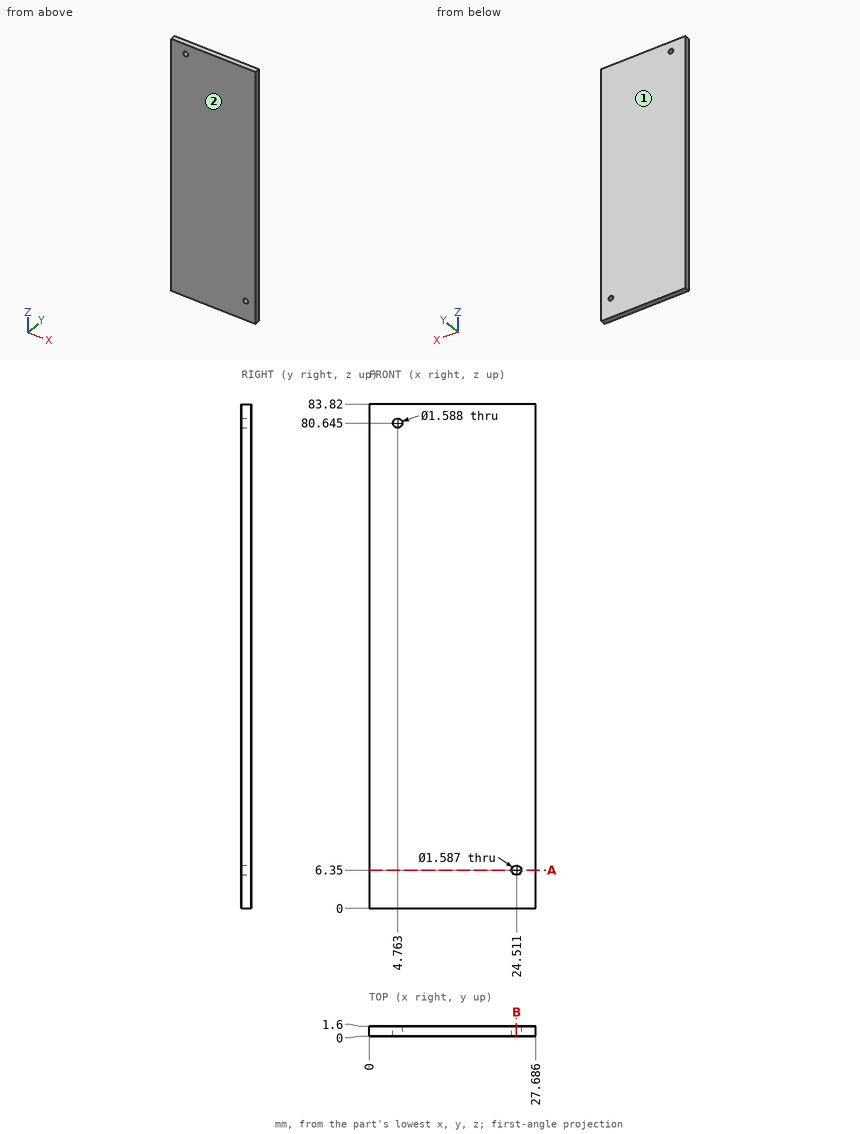
Here's the drawing with two shaded views (mm, measured from the low corner). I have some questions. Coordinates: 2 decimals unless noted, no trailing zeros. Write each loop counter-clockwise with the first axis right and the second up, starting at its lowest first coordinate (ties: lowest second). Pieces come first, ordered by that corner, then holes. Notation, with made-up numbers: M 5.25,-31 L 15.25,-31 A32 ccw 15.25,-5 Z; hole C -4,81.5 d4. An arc over 180 degrees is marked long. Answer as CSV lines item,"result". Start each with the question number.
1) I want a section at A-A, the plane z = 6.35. Please give me the cut outline in (x, y) (1 decimal).
2) We'd pull the mould along Y, two halves only. Please class the marked faces 1 and 2: +Y half, -Y half, draft (parallel to the pull), parting line (faces both ways), or undercut.
3) Please list where this line runs through material, in increasing order: line 1 (X direction, y = 0.2, z = 6) (1 decimal). Write a range as from..to.
4) I want a section at B-B, the plane x = 24.5. Please give me the cut outline in (y, z).
Data:
1,outline,"M 0,0 L 23.7,0 L 23.7,1.6 L 0,1.6 Z; M 25.3,0 L 27.7,0 L 27.7,1.6 L 25.3,1.6 Z"
2,face 1,"+Y half"
2,face 2,"-Y half"
3,line 1,"x = 0..23.8, 25.2..27.7"
4,outline,"M 0,0 L 1.6,0 L 1.6,5.56 L 0,5.56 Z; M 0,7.14 L 1.6,7.14 L 1.6,83.82 L 0,83.82 Z"
